```python
from build123d import *

# Parameters (mm, degrees)
SKICA1_R        = 20
VYSUNOUT1_DEPTH = 100
VYSUNOUT2_START = 20
VYSUNOUT2_DEPTH = 6


with BuildPart() as part:
    # Skica1 → Vysunout1 (new body)
    with BuildSketch(Plane(origin=(0, 0, 0), x_dir=(0, 0, -1), z_dir=(1, 0, 0))):
        Circle(SKICA1_R)
    extrude(amount=VYSUNOUT1_DEPTH)

    # Skica2 → Vysunout2 (cut)
    with BuildSketch(Plane(origin=(0, 0, 0), x_dir=(1, 0, 0), z_dir=(0, 1, 0)).offset(VYSUNOUT2_START)):
        with BuildLine():
            Line((31.593763982, 4.952572563), (35.592424808, 4.952572563))
            ThreePointArc((35.592424808, 4.952572563), (40.544997371, 0), (35.592424808, -4.952572563))
            Line((35.592424808, -4.952572563), (31.593763982, -4.952572563))
            ThreePointArc((31.593763982, -4.952572563), (26.64119142, 0), (31.593763982, 4.952572563))
        make_face()
    extrude(amount=-VYSUNOUT2_DEPTH, mode=Mode.SUBTRACT)


solid = part.part
```
CAD build for the part. Positions are in the model's coordinates, mm. A direction names the side the tool comes from. Round coordinates to 2 decimals unless told otherwise and drop trailing zeros. Order: outer loops, then holes, each group sorted by start corner. A loop starts at its lowest first (then second) coordinate and runs counter-clockwise, first axis right, second up.
Q1. Drop flat-ended pins along their axis: pin 1 (10 mm diameter, centred on x = 68, z = 15, fed in from +Y); pin 2 (3 mm diameter, centred on x = 33.5, y = 17.5, fed in from -Z); pin 3 (5 mm diameter, centred on x = 35, z = -1.5, fed in from +Y). Give the stop position or say it passes through.
Q2. Slice it at A-A (z = 0). Write the cut outline in (x, y) (3 decimals), and give its area (3 significant figures).
Q3. Two-plate mould, pull along X, no slides. Class faces 3 (the flat face through (34, 17, -4.953)), 4 (the flat face through (34, 14, 0)), 5 (the cylindrical face through (49.3, -19.524, 4.336)), 6 (the flat face through (100, 0, 0)): pulls with the +X half, pulls with the -X half, needs draft (parallel to the pull), parting line crosses it, or undercut.
Q4. Slice it at D-D (z = -7). Write the cut outline in (x, y) (3 decimals).
Q5. Slice it at C-C (y = -16.5). Write the cut outline in (x, z), and give its area (3 significant figures).
Q6. Slice it at B-B (x = 10.5). Write the cut outline in (y, z).
Q7. Which spindle directions (+Z, -Z, +X, -X, +Y, -Y) get a long thin tool onto all of the face, cutting with end or side? Do faces 1 (the flat face through (34, 17, 4.953)), 2 (the flat face through (0, 0, 0)). Say none if no direction does.
Q8. Wall check: L1, parallel to Y at x = 9, z = -0.5; L2, parallel to Z at x = 36.5, y = 16.5. Give the ranges that are in metal, low to high.
Results below:
1. pin 1: stops at y = 17.32
1. pin 2: stops at z = -12
1. pin 3: stops at y = 14
2. outline: (0, -20) - (100, -20) - (100, 20) - (40.545, 20) - (40.545, 14) - (26.641, 14) - (26.641, 20) - (0, 20) - close
2. area: 3,920 mm2
3. face 3: undercut
3. face 4: undercut
3. face 5: needs draft
3. face 6: pulls with the +X half
4. outline: (0, -18.735) - (100, -18.735) - (100, 18.735) - (0, 18.735) - close
5. outline: (0, -11.3) - (100, -11.3) - (100, 11.3) - (0, 11.3) - close
5. area: 2,260 mm2
6. outline: circle Ø40 at (0, 0)
7. face 1: +Y
7. face 2: +Z, -Z, -X, +Y, -Y
8. L1: y = -19.99 to 19.99
8. L2: z = -11.3 to -4.87, 4.87 to 11.3
